Could you check a few things on this model? Use its own coordinates, in mm. Face numbers are marked on the shaded views. Round coordinates to 2 decimals unless told otherwise and drop trailing zeros. Loops run counter-clockwise (first coordinate to the right, second up) from the corner with the lowest first, then second, coordinate; pieces in that order, holes last. Notation, with made-up numbers: (-40, -24) -> (-7, -24) arc R19 cw to (-7, 9) -> close; hole circle Ø8 at (-12, 68.25). An arc over 180 degrees is marked (long way). One line per item, written item: value.
from build123d import *

# Parameters (mm, degrees)
SKETCH1_R           = 50
SKETCH1_R_2         = 48.25
BOSS_EXTRUDE1_DEPTH = 100
SKETCH2_R           = 50
BOSS_EXTRUDE2_DEPTH = 1.5
SKETCH3_R           = 7.25
CUT_EXTRUDE1_DEPTH  = 2.5


with BuildPart() as part:
    # Sketch1 → Boss-Extrude1 (new body)
    with BuildSketch(Plane(origin=(0, 0, 0), x_dir=(1, 0, 0), z_dir=(0, 1, 0))):
        with Locations(Location((0, 0, 0), (0, 0, 270))):
            Circle(SKETCH1_R)
        with Locations(Location((0, 0, 0), (0, 0, 270))):
            Circle(SKETCH1_R_2, mode=Mode.SUBTRACT)
    extrude(amount=BOSS_EXTRUDE1_DEPTH)

    # Sketch2 → Boss-Extrude2 (add)
    with BuildSketch(Plane.XZ):
        with Locations(Location((0, 0, 0), (0, 0, 90))):
            Circle(SKETCH2_R)
    extrude(amount=-BOSS_EXTRUDE2_DEPTH)

    # Sketch3 → Cut-Extrude1 (cut)
    with BuildSketch(Plane.XZ):
        with Locations(Location((-20, 0, 0), (0, 0, 270))):
            Circle(SKETCH3_R)
        with Locations(Location((20, 0, 0), (0, 0, 270))):
            Circle(SKETCH3_R)
    extrude(amount=-CUT_EXTRUDE1_DEPTH, mode=Mode.SUBTRACT)


solid = part.part
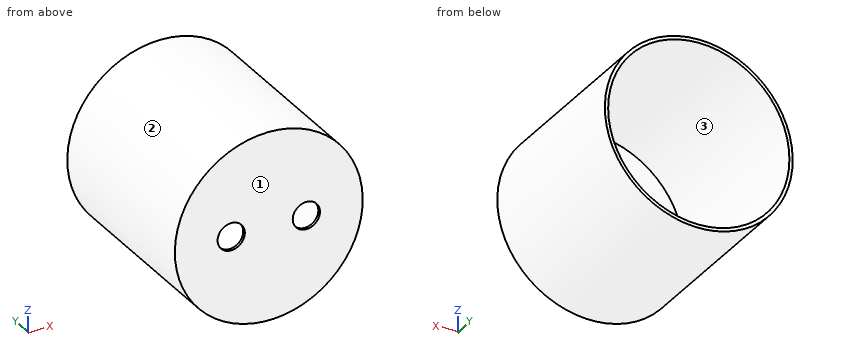
(1) If we section it at C-C, the plane x = -20: Please give me the cut outline in (y, z), then the cut area to 3 significant figures.
Recorded:
outline: (0, -45.83) -> (100, -45.83) -> (100, -43.91) -> (1.5, -43.91) -> (1.5, -7.25) -> (0, -7.25) -> close; (0, 7.25) -> (1.5, 7.25) -> (1.5, 43.91) -> (100, 43.91) -> (100, 45.83) -> (0, 45.83) -> close
area: 493 mm²
(2) Thinking about a two-plate mould opening in Z: for the marked faces 1, 2 and 3, which applies, released by +Z, released by -Z, zero draft, split by the parting line, or undercut?
Recorded:
face 1: zero draft
face 2: split by the parting line
face 3: undercut
(3) If we section it at B-B, the plane x = 0: Please give me the cut outline in (y, z).
Recorded:
outline: (0, -50) -> (100, -50) -> (100, -48.25) -> (1.5, -48.25) -> (1.5, 48.25) -> (100, 48.25) -> (100, 50) -> (0, 50) -> close
(4) I'm going to push flat-ended pins straight in: pin 1 Ø19 at (x, z) = (20, 0) entering from -Y; pin 2 Ø4 at (y, z) = (13, -14) entering from +X; pin 3 Ø1.5 at (y, z) = (34, 0) entering from +X; pin 4 Ø1.5 at (x, z) = (-14, 21.5) entering from +Y. Where does each tip first touch, or does it pass through?
Recorded:
pin 1: y = 0
pin 2: x = 48.54
pin 3: x = 50
pin 4: y = 1.5
(5) If I drill on L1, parallel to X at y = 1.05, z = 0; L2, parallel to X at y = 42.5, z = 0.5; L3, parallel to Z at x = -1, y = 72, over which ranges is the centre line in solid material (lowest first)?
Recorded:
L1: -50 to -27.25, -12.75 to 12.75, 27.25 to 50
L2: -50 to -48.25, 48.25 to 50
L3: -49.99 to -48.24, 48.24 to 49.99
(6) If we section it at D-D, the plane z = -20: Please give me the cut outline in (x, y), then the cut area to 3 significant figures.
Recorded:
outline: (-45.83, 0) -> (45.83, 0) -> (45.83, 100) -> (43.91, 100) -> (43.91, 1.5) -> (-43.91, 1.5) -> (-43.91, 100) -> (-45.83, 100) -> close
area: 515 mm²
(7) If we section it at A-A, the plane z = 0: Please give me the cut outline in (x, y), then the cut area to 3 significant figures.
Recorded:
outline: (-50, 0) -> (-27.25, 0) -> (-27.25, 1.5) -> (-48.25, 1.5) -> (-48.25, 100) -> (-50, 100) -> close; (-12.75, 0) -> (12.75, 0) -> (12.75, 1.5) -> (-12.75, 1.5) -> close; (27.25, 0) -> (50, 0) -> (50, 100) -> (48.25, 100) -> (48.25, 1.5) -> (27.25, 1.5) -> close
area: 451 mm²
